from build123d import *

# Parameters (mm, degrees)
BOSS_EXTRUDE1_DEPTH     = 36
SKETCH2_R               = 1.9
CUT_EXTRUDE1_DEPTH      = 39.543989963
CUT_EXTRUDE2_DEPTH      = 39.543989963
CUT_EXTRUDE2_DEPTH_BACK = 39.543989963
SKETCH3_W               = 8.124276203
SKETCH3_H               = 16.8


with BuildPart() as part:
    # Sketch1 → Boss-Extrude1 (new body)
    with BuildSketch(Plane.XY):
        with BuildLine():
            Line((0, 0), (0, 0.6))
            Line((0, 0.6), (-11.712138102, 0.6))
            ThreePointArc((-11.712138102, 0.6), (-12.215259426, 2.784102961), (-10.807304622, 1.040227943))
            Line((-10.807304622, 1.040227943), (-10.335217589, 0.669912086))
            ThreePointArc((-10.335217589, 0.669912086), (-12.477757508, 3.32363494), (-11.712138102, 0))
            Line((-11.712138102, 0), (0, 0))
        make_face()
    extrude(amount=BOSS_EXTRUDE1_DEPTH)

    # Sketch2 → Cut-Extrude1 (cut, through all)
    with BuildSketch(Plane(origin=(0, 0.6, 0), x_dir=(1, 0, 0), z_dir=(0, 1, 0))):
        with Locations(Location((-4.5, -5, 0), (0, 0, 180))):
            Circle(SKETCH2_R)
        with Locations(Location((-4.5, -31, 0), (0, 0, 180))):
            Circle(SKETCH2_R)
    extrude(amount=-CUT_EXTRUDE1_DEPTH, mode=Mode.SUBTRACT)

    # Sketch3 → Cut-Extrude2 (cut, two sides: drawn at the far end of the back side and taken through both)
    with BuildSketch(Plane(origin=(0, 0.6, 0), x_dir=(1, 0, 0), z_dir=(0, 1, 0)).offset(-CUT_EXTRUDE2_DEPTH_BACK)):
        with Locations((-13.462138101, -18)):
            Rectangle(SKETCH3_W, SKETCH3_H)
    extrude(amount=CUT_EXTRUDE2_DEPTH + CUT_EXTRUDE2_DEPTH_BACK, mode=Mode.SUBTRACT)


solid = part.part
Input: part model. Units: mm. Frame: model coordinates. Coordinates: 2 decimals unless noted, no trailing zeros. Loops run counter-clockwise (first coordinate to the right, second up) from the corner with the lowest first, then second, coordinate; pieces in that order, holes last.
Q1. Draft query along X for faces 1 (the face through (-4.253, 0.304, 32.884)), 2 (the face through (-12.42, 3.35, 4.73)), 3 (the face through (-6, 0, 18)). Return one class per face: +X half, -X half, draft (parallel to the pull), parting line (faces both ways), or undercut.
Q2. Cut plane A-A (z = 5). Output: boundary loops of the cut face in (x, y), then the cut area to 3 significant figures.
Q3. Material intervals for line 1 (Z direction, x = -4.5, y = 0.45); line 2 (Z direction, x = -10.75, y = 0.5); line 3 (X direction, y = 1.75, z = 7.25), sorted ascending.
Q4. Cut plane D-D (x = -2). Output: boundary loops of the cut face in (y, z).
Q5. Cut plane B-B (y = 1.75). Output: boundary loops of the cut face in (x, z).
Q6. Contact query for flat-ended pins moving along their axis: pin 1 (1 mm diameter, centred on x = -6, z = 27, fed in from +Y); pin 2 (3.5 mm diameter, centred on x = -8.5, z = 26, fed in from +Y); pin 3 (0.5 mm diameter, centred on y = 0.5, z = 18.5, fed in from -X). Output: stop coordinate, or through.
Q7. Cut plane C-C (z = 32). Output: boundary loops of the cut face in (x, y), then the cut area to 3 significant figures.
Working result:
1. face 1: undercut
1. face 2: parting line
1. face 3: draft
2. outline: (-11.71, 0) - (-6.4, 0) - (-6.4, 0.6) - (-11.71, 0.6) arc R1.15 cw (long way) to (-10.81, 1.04) - (-10.34, 0.67) arc R1.75 ccw (long way) to start; (-2.6, 0) - (0, 0) - (0, 0.6) - (-2.6, 0.6) - close
2. area: 9.43 mm2
3. line 1: z = 0 to 3.1, 6.9 to 29.1, 32.9 to 36
3. line 2: z = 0 to 9.6, 26.4 to 36
3. line 3: x = -13.46 to -12.86, -10.56 to -9.96
4. outline: (0, 0) - (0.6, 0) - (0.6, 36) - (0, 36) - close
5. outline: (-13.46, 0) - (-12.86, 0) - (-12.86, 9.6) - (-13.46, 9.6) - close; (-13.46, 26.4) - (-12.86, 26.4) - (-12.86, 36) - (-13.46, 36) - close; (-10.56, 0) - (-9.96, 0) - (-9.96, 9.6) - (-10.56, 9.6) - close; (-10.56, 26.4) - (-9.96, 26.4) - (-9.96, 36) - (-10.56, 36) - close
6. pin 1: stops at y = 0.6
6. pin 2: stops at y = 2.64
6. pin 3: stops at x = -9.4
7. outline: (-11.71, 0) - (-6.12, 0) - (-6.12, 0.6) - (-11.71, 0.6) arc R1.15 cw (long way) to (-10.81, 1.04) - (-10.34, 0.67) arc R1.75 ccw (long way) to start; (-2.88, 0) - (0, 0) - (0, 0.6) - (-2.88, 0.6) - close
7. area: 9.77 mm2
